from build123d import *

# Parameters (mm, degrees)
SKETCH1_R           = 29.55371142
BOSS_EXTRUDE1_DEPTH = 11.355
CUT_EXTRUDE1_DEPTH  = 9.998813
CUT_EXTRUDE5_DEPTH  = 10
CUT_EXTRUDE6_DEPTH  = 9.999998
CUT_EXTRUDE7_DEPTH  = 10
FILLET1_R           = 4


# Read off the part's stored shape, not the designer's step: Surface-Imported1
with BuildPart() as part:
    # Sketch1 → Boss-Extrude1 (new body)
    with BuildSketch(Plane(origin=(0, 0, 0), x_dir=(1, 0, 0), z_dir=(0, 1, 0))):
        with BuildLine():
            Line((16.123584474, 0), (63.875229096, 0))
            ThreePointArc((63.875229096, 0), (68.091521161, -1.20125885), (71.041598686, -4.444279694))
            ThreePointArc((71.041598686, -4.444279694), (72.928335493, -7.070478077), (75.554533876, -8.957214884))
            ThreePointArc((75.554533876, -8.957214884), (78.79755472, -11.907292409), (79.99881357, -16.123584474))
            Line((79.99881357, -16.123584474), (79.99881357, -63.876413738))
            ThreePointArc((79.99881357, -63.876413738), (78.79755472, -68.092705803), (75.554533876, -71.042783328))
            ThreePointArc((75.554533876, -71.042783328), (72.928335493, -72.929520135), (71.041598686, -75.555718518))
            ThreePointArc((71.041598686, -75.555718518), (68.091521161, -78.798739362), (63.875229096, -79.999998212))
            Line((63.875229096, -79.999998212), (16.123584474, -79.999998212))
            ThreePointArc((16.123584474, -79.999998212), (11.907292409, -78.798739362), (8.957214884, -75.555718518))
            ThreePointArc((8.957214884, -75.555718518), (7.070478077, -72.929520135), (4.444279694, -71.042783328))
            ThreePointArc((4.444279694, -71.042783328), (1.20125885, -68.092705803), (0, -63.876413738))
            Line((0, -63.876413738), (0, -16.123584474))
            ThreePointArc((0, -16.123584474), (1.20125885, -11.907292409), (4.444279694, -8.957214884))
            ThreePointArc((4.444279694, -8.957214884), (7.070478077, -7.070478077), (8.957214884, -4.444279694))
            ThreePointArc((8.957214884, -4.444279694), (11.907292409, -1.20125885), (16.123584474, 0))
        make_face()
        with Locations(Location((39.999406785, -39.999999106, 0), (0, 0, 270))):
            Circle(SKETCH1_R, mode=Mode.SUBTRACT)
    extrude(amount=BOSS_EXTRUDE1_DEPTH)

    # Sketch2 → Cut-Extrude1 (cut)
    with BuildSketch(Plane(origin=(79.99881357, 0, 0), x_dir=(0, 0, -1), z_dir=(1, 0, 0))):
        with BuildLine():
            Line((-56.770510972, 11.581630446), (-23.229489103, 11.581630446))
            ThreePointArc((-23.229489103, 11.581630446), (-40.000000037, 4.081632348), (-56.770510972, 11.581630446))
        make_face()
    extrude(amount=-CUT_EXTRUDE1_DEPTH, mode=Mode.SUBTRACT)

    # Sketch3 → Cut-Extrude5 (cut)
    with BuildSketch(Plane.ZY):
        with BuildLine():
            Line((23.229489103, 11.581630446), (56.770510972, 11.581630446))
            ThreePointArc((56.770510972, 11.581630446), (40.000000037, 4.081630803), (23.229489103, 11.581630446))
        make_face()
    extrude(amount=-CUT_EXTRUDE5_DEPTH, mode=Mode.SUBTRACT)

    # Sketch4 → Cut-Extrude6 (cut)
    with BuildSketch(Plane.XY.offset(79.999998212)):
        with BuildLine():
            Line((23.229489103, 11.581630446), (56.770510972, 11.581630446))
            ThreePointArc((56.770510972, 11.581630446), (40.000000037, 4.081632696), (23.229489103, 11.581630446))
        make_face()
    extrude(amount=-CUT_EXTRUDE6_DEPTH, mode=Mode.SUBTRACT)

    # Sketch5 → Cut-Extrude7 (cut)
    with BuildSketch(Plane(origin=(0, 0, 0), x_dir=(-1, 0, 0), z_dir=(0, 0, -1))):
        with BuildLine():
            Line((-56.770510972, 11.581630446), (-23.229489103, 11.581630446))
            ThreePointArc((-23.229489103, 11.581630446), (-40.000000037, 4.081631894), (-56.770510972, 11.581630446))
        make_face()
    extrude(amount=-CUT_EXTRUDE7_DEPTH, mode=Mode.SUBTRACT)

    # Fillet1
    fillet1_edges = [part.edges().sort_by_distance(p)[0] for p in [
        (7.070478077, 0, 7.070478077),
        (11.907292409, 0, 1.20125885),
        (39.999406785, 0, 0),
        (68.091521161, 0, 1.20125885),
        (72.928335493, 0, 7.070478077),
        (78.79755472, 0, 11.907292409),
        (79.99881357, 0, 39.999999106),
        (78.79755472, 0, 68.092705803),
        (72.928335493, 0, 72.929520135),
        (68.091521161, 0, 78.798739362),
        (39.999406785, 0, 79.999998212),
        (11.907292409, 0, 78.798739362),
        (7.070478077, 0, 72.929520135),
        (1.20125885, 0, 68.092705803),
        (0, 0, 39.999999106),
        (1.20125885, 0, 11.907292409),
        (39.999406785, 0, 10.446287686),
    ]]
    fillet(fillet1_edges, radius=FILLET1_R)


solid = part.part
Could you check a few things on this model? Use its own coordinates, in mm. A direction names the side the tool comes from. Round coordinates to 2 decimals unless told otherwise and drop trailing zeros. Put each result on its own line as item: value. Start each with the question number.
(1) Thinking about a two-plate mould opening in Z: for faces 1 (the flat face through (45.6, 4.4, 80)), 2 (the cylindrical face through (75.069, 4.083, 39.739)), 3 (the cylindrical face through (39.739, 4.083, 4.93)), which applies, released by +Z, released by -Z, zero draft, split by the parting line, or undercut?
(2) For faces 4 (the flat face through (70, 9, 40)), 5 (the flat face through (40, 9, 10)), 6 (the flat face through (40, 9, 70)), which set-ups out of +Z, -Z, +X, -X, +Y, -Y let a thin tool reach every point of the face, with its end or its side?
(3) Will these pins go through, and if not, where does the flat tip stop? pin 1 (3 mm diameter, centred on x = 66, y = 3, fed in from +Z); pin 2 (2 mm diameter, centred on x = 41.5, y = 8.5, fed in from -Z); pin 3 (6 mm diameter, centred on y = 3, z = 18, fed in from +X); pin 4 (3 mm diameter, centred on x = 70, y = 6, fed in from +Z).
(4) I need wall thicknesses on probe 1 along X at (y, z) = (8.5, 40); probe 2 along X at (y, z) = (6.25, 39); probe 3 along Z at (x, y) = (74.5, 9.75). Which ranges of each line are inside material? Lowest first, please.
Here are the results:
1. face 1: released by +Z
1. face 2: undercut
1. face 3: zero draft
2. face 4: +X, +Y
2. face 5: -Z, +Y
2. face 6: +Z, +Y
3. pin 1: stops at z = 79.95
3. pin 2: stops at z = 10
3. pin 3: stops at x = 80
3. pin 4: stops at z = 78.53
4. probe 1: x = 10 to 10.45, 69.55 to 70
4. probe 2: x = 10 to 10.46, 69.54 to 70
4. probe 3: z = 8.35 to 25.07, 54.93 to 71.65
